```python
from build123d import *

# Parameters (mm, degrees)
SKETCH_1_W          = 30
SKETCH_1_H          = 61.5
EXTRUDE_1_DEPTH     = 5
SKETCH_2_R          = 1.75
SKETCH_2_W          = 21
SKETCH_2_H          = 41
CUT_EXTRUDE_1_DEPTH = 6
SKETCH_3_W          = 30
SKETCH_3_H          = 40
EXTRUDE_2_DEPTH     = 5
SKETCH_4_R          = 1.75
CUT_EXTRUDE_2_DEPTH = 62.5
SKETCH_5_W          = 10
SKETCH_5_H          = 12
EXTRUDE_3_DEPTH     = 2.3
SKETCH_6_W          = 30
SKETCH_6_H          = 12
EXTRUDE_4_DEPTH     = 4
EXTRUDE_5_DEPTH     = 4.5
FILLET_1_R          = 5
SKETCH_8_W          = 21
SKETCH_8_H          = 6
CUT_EXTRUDE_3_DEPTH = 10


with BuildPart() as part:
    # ｽｹｯﾁ1 → ﾎﾞｽ - 押し出し1 (new body)
    with BuildSketch(Plane.XY):
        with Locations((15, 30.75)):
            Rectangle(SKETCH_1_W, SKETCH_1_H)
    extrude(amount=EXTRUDE_1_DEPTH)

    # ｽｹｯﾁ2 → ｶｯﾄ - 押し出し1 (cut, through all)
    with BuildSketch(Plane.XY.offset(5)):
        with Locations((10, 3.5)):
            Circle(SKETCH_2_R)
        with Locations((20, 3.5)):
            Circle(SKETCH_2_R)
        with Locations((10, 53)):
            Circle(SKETCH_2_R)
        with Locations((20, 53)):
            Circle(SKETCH_2_R)
        with Locations((15, 28.2)):
            Rectangle(SKETCH_2_W, SKETCH_2_H)
    extrude(amount=-CUT_EXTRUDE_1_DEPTH, mode=Mode.SUBTRACT)

    # ｽｹｯﾁ3 → ﾎﾞｽ - 押し出し2 (add)
    with BuildSketch(Plane(origin=(0, 61.5, 0), x_dir=(1, 0, 0), z_dir=(0, 1, 0))):
        with Locations((15, 20)):
            Rectangle(SKETCH_3_W, SKETCH_3_H)
    extrude(amount=-EXTRUDE_2_DEPTH)

    # ｽｹｯﾁ4 → ｶｯﾄ - 押し出し2 (cut, through all)
    with BuildSketch(Plane(origin=(0, 61.5, 0), x_dir=(1, 0, 0), z_dir=(0, 1, 0))):
        with Locations((5, 25)):
            Circle(SKETCH_4_R)
        with Locations((25, 25)):
            Circle(SKETCH_4_R)
    extrude(amount=-CUT_EXTRUDE_2_DEPTH, mode=Mode.SUBTRACT)

    # ｽｹｯﾁ5 → ﾎﾞｽ - 押し出し3 (add)
    with BuildSketch(Plane.XZ.offset(-56.5)):
        with Locations((5, -25)):
            Rectangle(SKETCH_5_W, SKETCH_5_H)
        Polygon((5, -28.6), (8.117691454, -26.8), (8.117691454, -23.2), (5, -21.4), (1.882308546, -23.2), (1.882308546, -26.8), align=None, mode=Mode.SUBTRACT)
        with Locations((25, -25)):
            Rectangle(SKETCH_5_W, SKETCH_5_H)
        Polygon((28.117691454, -26.8), (25, -28.6), (21.882308546, -26.8), (21.882308546, -23.2), (25, -21.4), (28.117691454, -23.2), align=None, mode=Mode.SUBTRACT)
    extrude(amount=EXTRUDE_3_DEPTH)

    # ｽｹｯﾁ6 → ﾎﾞｽ - 押し出し4 (add)
    with BuildSketch(Plane(origin=(0, 61.5, 0), x_dir=(1, 0, 0), z_dir=(0, 1, 0))):
        with Locations((15, 1)):
            Rectangle(SKETCH_6_W, SKETCH_6_H)
    extrude(amount=EXTRUDE_4_DEPTH)

    # ｽｹｯﾁ7 → ﾎﾞｽ - 押し出し5 (add)
    with BuildSketch(Plane(origin=(30, 0, 0), x_dir=(0, 0, -1), z_dir=(1, 0, 0))):
        Polygon((40, 56.5), (40, 39.5), (0, 9.822580645), (0, 21.5), (31, 44.5), (31, 56.5), align=None)
    extrude_5 = extrude(amount=-EXTRUDE_5_DEPTH)

    # ﾐﾗｰ1: ﾎﾞｽ - 押し出し5 across plane
    add(extrude_5.mirror(Plane.ZY.offset(-15)))

    # ﾌｨﾚｯﾄ1
    fillet_1_edges = [part.edges().sort_by_distance(p)[0] for p in [
        (30, 0, 2.5),
        (0, 0, 2.5),
    ]]
    fillet(fillet_1_edges, radius=FILLET_1_R)

    # ｽｹｯﾁ8 → ｶｯﾄ - 押し出し3 (cut, through all)
    with BuildSketch(Plane.XZ.offset(-56.5)):
        with Locations((15, -37)):
            Rectangle(SKETCH_8_W, SKETCH_8_H)
    extrude(amount=-CUT_EXTRUDE_3_DEPTH, mode=Mode.SUBTRACT)


solid = part.part
```
Here's how the part is built. I have some questions about the finished solid (model axes, mm). A direction names the side the tool comes from. Round coordinates to 2 decimals unless told otherwise and drop trailing zeros. Order: outer loops, then holes, each group sorted by start corner. A loop starts at its lowest first (then second) coordinate and runs counter-clockwise, first axis right, second up. Notation, with made-up numbers: (-14.5, 19.5) -> (29.5, 19.5) arc R16 ccw to (29.5, 44.5) -> close; hole circle Ø9 at (-39.5, -5.75). An arc over 180 degrees is marked (long way). Use a Markdown table: item, result. Add a question column.
(1) For faces 5 (the face through (15, 7.7, 3)), 6 (the face through (15, 56.5, -13)), 7 (the face through (2.218, 32.839, -15.283)), 8 (the face through (8.118, 55, -25)), which set-ups out of +Z, -Z, +X, -X, +Y, -Y let a thin tool reach every point of the face, with its end or its side?
(2) Suppose I cut it at B-B, the plane z = -5.5. Please give me the cut outline in (x, y), and give its area (3 significant figures).
(3) For pin 1 Ø3 at (x, z) = (5, -25) entering from +Y; pin 2 Ø1.8 at (y, z) = (55, -23) entering from -X; pin 3 Ø2 at (x, y) = (20, 53) entering from +Z; pin 4 Ø5.5 at (x, y) = (20, 3.5) entering from -Z, each with a flat end and sliding along its axis, tell me the tip position at first contact or that it passes through.
(4) Suppose I cut it at C-C, the plane y = 17.5. Please give me the cut outline in (x, z), and give its area (3 significant figures).
(5) Suppose I cut it at A-A, the plane y = 53. Please give me the cut outline in (x, z), and give its area (3 significant figures).
(6) If we mould it in two halves opening along Y, with no side actions, what happens to faces 1 (the face through (27.78, 24.87, -20.28)), 2 (the face through (28.118, 55, -25)), 3 (the face through (6.54, 55.37, -27.71)), 4 (the face through (15, 61.5, -20))? For each: released by +Y, released by -Y, zero draft, split by the parting line, or undercut.
(7) Suppose I cut it at D-D, the plane z = -25. Count the separate pieces of the cut face and the enclosed holes in it, and give its area (3 significant figures).
(8) I need wall thicknesses on line 1 along Y through (x, z) = (20, 2.95); line 2 along X through (y, z) = (58.35, -25); line 3 along Z through (x, y) = (5, 59.65). Which ranges of each line are inside material? Lowest first, please.
Verdict:
| question | item | result |
|---|---|---|
| 1 | face 5 | +Z, -Z |
| 1 | face 6 | none |
| 1 | face 7 | +X, -X |
| 1 | face 8 | -Y |
| 2 | outline | (0, 13.9) -> (4.5, 13.9) -> (4.5, 25.58) -> (0, 25.58) -> close; (0, 56.5) -> (30, 56.5) -> (30, 65.5) -> (0, 65.5) -> close; (25.5, 13.9) -> (30, 13.9) -> (30, 25.58) -> (25.5, 25.58) -> close |
| 2 | area | 375 mm2 |
| 3 | pin 1 | y = 41.1 |
| 3 | pin 2 | x = 0 |
| 3 | pin 3 | through |
| 3 | pin 4 | z = 0 |
| 4 | outline | (0, -10.35) -> (4.5, -10.35) -> (4.5, 5) -> (0, 5) -> close; (25.5, -10.35) -> (30, -10.35) -> (30, 5) -> (25.5, 5) -> close |
| 4 | area | 138 mm2 |
| 5 | outline | (0, -40) -> (4.5, -40) -> (4.5, -31) -> (0, -31) -> close; (0, 0) -> (8.25, 0) -> (8.25, 5) -> (0, 5) -> close; (11.75, 0) -> (18.25, 0) -> (18.25, 5) -> (11.75, 5) -> close; (21.75, 0) -> (30, 0) -> (30, 5) -> (21.75, 5) -> close; (25.5, -40) -> (30, -40) -> (30, -31) -> (25.5, -31) -> close |
| 5 | area | 196 mm2 |
| 6 | face 1 | released by -Y |
| 6 | face 2 | undercut |
| 6 | face 3 | zero draft |
| 6 | face 4 | released by +Y |
| 7 | separate pieces | 5 |
| 7 | enclosed holes | 0 |
| 7 | area | 237 mm2 |
| 8 | line 1 | 0 to 1.75, 5.25 to 7.7, 48.7 to 51.25, 54.75 to 65.5 |
| 8 | line 2 | 0 to 3.25, 6.75 to 23.25, 26.75 to 30 |
| 8 | line 3 | -34 to -26.75, -23.25 to 5 |
